Could you check a few things on this model? Use its own coordinates, in mm. Face numbers are marked on the shaded views. A direction names the side the tool comes from. Coordinates: 2 decimals unless noted, no trailing zeros. Order: outer loops, then holes, each group sorted by start corner. A loop starts at its lowest first (then second) coordinate and runs counter-clockwise, first axis right, second up. Notation, with made-up numbers: (22, 21) -> (57, 21) arc R21 ccw to (57, 53) -> close; hole circle Ø2 at (-35, 18.25). An arc over 180 degrees is marked (long way). Use a Markdown table: item, result. Add a question column.
1) Which directions (+Z, -Z, +X, -X, +Y, -Y) give clear straight access to the entire face, cutting with the end or side of a thin tool? Please do the marked faces 1, 2 and 3.
2) If we section it at A-A (y = -10): Write out the boundary of the cut face in (x, z).
3) Will these pins go through, and if not, where does the flat tip stop? pin 1 Ø3.5 at (x, y) = (14.5, -2) entering from -Z; pin 2 Ø6 at (y, z) = (-6.5, 4.5) entering from -X; pin 3 Ø4.5 at (x, y) = (-19, -16) entering from +Z.
4) If we section it at B-B (z = 29.5): Write out the boundary of the cut face in (x, y).
5) If I drill on L1, parallel to Z at x = 20.5, y = -12; L2, parallel to X at y = -11.25, z = 9.5; L3, parallel to X at y = -13.25, z = 8, over which ranges is the centre line in solid material (lowest first)? Write a range as [from, to].
6) If we section it at C-C (y = -14.5): Write out the boundary of the cut face in (x, z).
```python
from build123d import *

# Parameters (mm, degrees)
F1_DEPTH  = 25
F2_R      = 5
F4_DEPTH  = 25
F5_R      = 4.586738227
F6_DEPTH  = 8.5901785642
F7_R      = 3.6228791996
F8_DEPTH  = 28.0857570469
F9_R      = 3.1821948937
F10_DEPTH = 44.3071853369


with BuildPart() as f1:
    # F0 (on Front) → F1 (new body)
    with BuildSketch(Plane.XZ):
        Polygon((-36.51381284, 22.3948657513), (0, 0), (23.6873179674, 22.3948657513), align=None)
    extrude(amount=F1_DEPTH)

    # F2
    f2_edges = [f1.edges().sort_by_distance(p)[0] for p in [
        (11.843659, -25, 11.197433),
        (11.843659, 0, 11.197433),
        (-18.256906, -25, 11.197433),
        (-6.413247, 0, 22.394866),
        (-6.413247, -25, 22.394866),
    ]]
    fillet(f2_edges, radius=F2_R)

    # F3 (on Front) → F4 (join)
    with BuildSketch(Plane.XZ):
        with BuildLine():
            Line((-8.0289142206, 22.2887210548), (23.4841555357, 22.2887210548))
            Line((23.4841555357, 22.2887210548), (23.4841555357, 41.8256605239))
            ThreePointArc((23.4841555357, 41.8256605239), (10.5100013982, 27.5692125926), (-8.0289142206, 22.2887210548))
        make_face()
    extrude(amount=F4_DEPTH)

    # F5 (on face) → F6 (join)
    with BuildSketch(Plane(origin=(0, 0, 0), x_dir=(0.7266530358, 0, 0.6870046329), z_dir=(0.6870046329, 0, -0.7266530358))):
        with Locations((16.2989190171, 12.5)):
            Circle(F5_R)
    extrude(amount=F6_DEPTH)

    # F7 (on face) → F8 (join)
    with BuildSketch(Plane(origin=(5.9014924708, 0, -6.2420793316), x_dir=(0.7266530358, 0, 0.6870046329), z_dir=(0.6870046329, 0, -0.7266530358))):
        with Locations((16.2989190171, 12.5)):
            Circle(F7_R)
    extrude(amount=-F8_DEPTH)

    # F9 (on face) → F10 (cut)
    with BuildSketch(Plane(origin=(-13.3935527382, 0, 14.1665212888), x_dir=(0.7266530358, 0, 0.6870046329), z_dir=(-0.6870046329, 0, 0.7266530358))):
        with Locations((16.2989190171, -12.5)):
            Circle(F9_R)
    extrude(amount=-F10_DEPTH, mode=Mode.SUBTRACT)


solid = f1.part
```
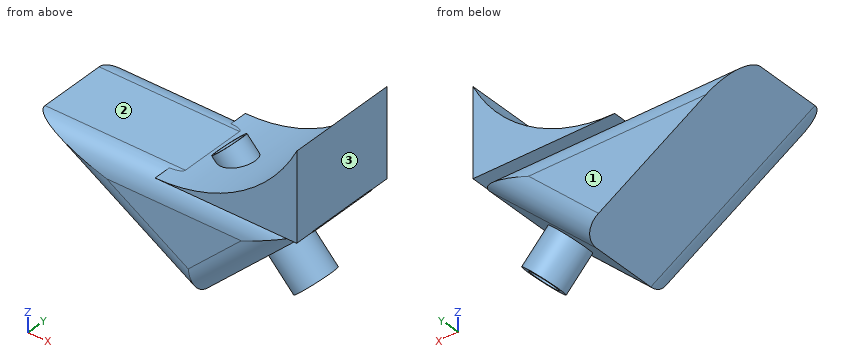
Answer sheet:
| question | item | result |
|---|---|---|
| 1 | face 1 | +Z, -Z, +X, -X, +Y |
| 1 | face 2 | +Z, -X, +Y, -Y |
| 1 | face 3 | +Z, +X, +Y, -Y |
| 2 | outline | (-36.51, 22.39) -> (0, 0) -> (9.05, 8.56) -> (14.95, 2.31) -> (16.31, 3.6) -> (-2.98, 24.01) -> (-3.46, 23.56) -> (-2.64, 22.7) arc R35.18 cw to (-5.3, 22.39) -> close; (-0.12, 26.72) -> (19.18, 6.31) -> (20.54, 7.6) -> (14.64, 13.84) -> (23.69, 22.39) -> (23.48, 22.39) -> (23.48, 41.83) arc R35.18 cw to (3.22, 24.14) -> (0.36, 27.17) -> close |
| 3 | pin 1 | z = 12.92 |
| 3 | pin 2 | x = -12.23 |
| 3 | pin 3 | z = 22.39 |
| 4 | outline | (13.31, -25) -> (23.48, -25) -> (23.48, 0) -> (13.31, 0) -> close |
| 5 | L1 | [7.56, 8.68], [19.38, 36.88] |
| 5 | L2 | [-15.49, 9.42], [17.48, 19.52] |
| 5 | L3 | [-13.04, 8.46], [8.64, 10.61], [19.12, 20.97] |
| 6 | outline | (-36.51, 22.39) -> (0, 0) -> (8.84, 8.36) -> (14.75, 2.12) -> (15.95, 3.25) -> (-3.35, 23.66) -> (-3.74, 23.29) -> (-3.12, 22.63) arc R35.18 cw to (-5.3, 22.39) -> close; (0.25, 27.06) -> (19.54, 6.66) -> (20.74, 7.79) -> (14.84, 14.03) -> (23.69, 22.39) -> (23.48, 22.39) -> (23.48, 41.83) arc R35.18 cw to (3.63, 24.28) -> (0.65, 27.44) -> close |
